Design review of the part built by this model. Coordinates are the model's own, in mm. Face numbers are marked on the shaded views. A direction names the side the tool comes from. Coordinates: 2 decimals unless noted, no trailing zeros. Loops run counter-clockwise (first coordinate to the right, second up) from the corner with the lowest first, then second, coordinate; pieces in that order, holes last. Notation, with made-up numbers: M 81.25,-26.5 L 128.25,-26.5 A30 cw 128.25,2.5 Z; hole C -39.5,48.5 d1. An arc over 180 degrees is marked long. One line per item, written item: value.
Autodesk Fusion 360 part; units mm, degrees
sketch "Sketch1" plane through (0, 0, 0) normal (0, 1, 0) x (1, 0, 0)
  line L0 (60, 15) -> (-60, 15)
  line L1 (-60, 15) -> (-60, -15)
  line L2 (-60, -15) -> (60, -15)
  line L3 (60, -15) -> (60, 15)
  line L4 (60, 15) -> (-60, -15) construction
  line L5 (-60, 15) -> (60, -15) construction
  line L6 (0, -15) -> (0, -60)
  line L7 (40, -15) -> (-40, -15)
  line L8 (-40, -15) -> (-40, -60)
  line L9 (-40, -60) -> (40, -60)
  line L10 (40, -60) -> (40, -15)
  line L11 (40, -15) -> (-40, -60) construction
  line L12 (-40, -15) -> (40, -60) construction
  line L13 (20, -40) -> (-20, -40)
  line L14 (-20, -40) -> (-20, -80)
  line L15 (-20, -80) -> (20, -80)
  line L16 (20, -80) -> (20, -40)
  line L17 (20, -40) -> (-20, -80) construction
  line L18 (-20, -40) -> (20, -80) construction
  point P0 (0, -37.5)
  point P1 (0, -60)
  dimension "d1" = 120
  dimension "d2" = 30
  dimension "d3" = 45
  dimension "d4" = 80
  dimension "d5" = 40
  dimension "d6" = 40
extrude "Extrude1" add sketch "Sketch1" along normal blind 80 contours L0 L1 L2 L3 L7 | L2 L6 L7 L9 L10 L13 L16 | L2 L6 L7 L8 L9 L13 L14
sketch "Sketch2" plane through (40, 0, 0) normal (1, 0, 0) x (0, 1, 0)
  line L0 (0, 60) -> (0, 15)
  line L1 (0, 15) -> (80, 15)
  line L2 (80, 15) -> (80, 60)
  line L3 (80, 60) -> (0, 60)
  circle A0 centre (40, 60) radius 15
  dimension "d9" = 30
extrude "Extrude2" cut sketch "Sketch2" against normal blind 100 contours L3 A0 | L3 A0
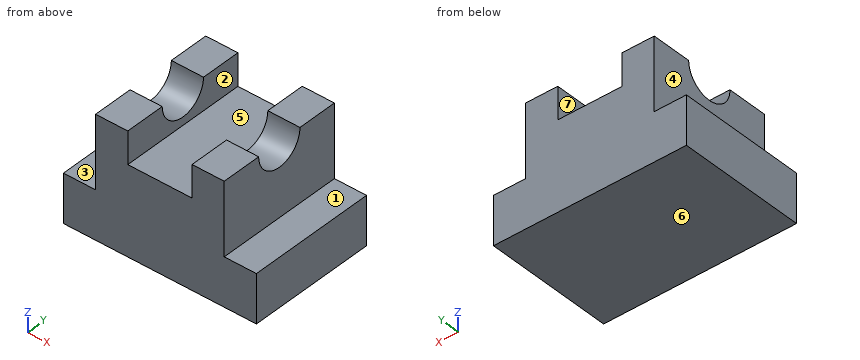
(1) We need section C-C on x = -6.5. State the section outline as (y, z) points.
Reply:
outline: M 0,-15 L 80,-15 L 80,40 L 0,40 Z
(2) Tool access review of the marked faces 1, 2 and 3: name each direction out of +Z, -Z, +X, -X, +Y, -Y from which nothing blocks a thin tool from reaching the whole face with its end or side.
Reply:
face 1: +Z, +X, +Y, -Y
face 2: +Z, +Y, -Y
face 3: +Z, -X, +Y, -Y
(3) Insertion check: pin 1 (10 mm diameter, centred on y = 51, z = 49, fed in from +X); pin 2 (22 mm diameter, centred on y = 31, z = 49, fed in from -X); pin 3 (3 mm diameter, centred on x = -9.5, y = 40, fed in from +Z). Each pin has a flat end and moves straight along its axis. Give the tip position at first contact, or say it passes through.
Reply:
pin 1: stops at x = 40
pin 2: stops at x = -40
pin 3: stops at z = 40
(4) Mouldability with a two-part tool opening along X and no side actions: class the marked faces 4, 5, 6 and 7 as released by +X, released by -X, zero draft, split by the parting line, or undercut.
Reply:
face 4: released by -X
face 5: undercut
face 6: zero draft
face 7: undercut
(5) We need section A-A on z = 50. State the section outline as (x, y) points.
Reply:
outline: M -40,0 L -20,0 L -20,28.82 L -40,28.82 Z; M -40,51.18 L -20,51.18 L -20,80 L -40,80 Z; M 20,0 L 40,0 L 40,28.82 L 20,28.82 Z; M 20,51.18 L 40,51.18 L 40,80 L 20,80 Z
(6) To check wall thickness, follow line 1 along X through (y, z) = (23, 50); line 2 along Z through (x, y) = (-44.5, 14); line 3 along X through (y, z) = (47, 30). State the ranges of each line that lie inside material, in increasing order. Write a range as [from, to].
Reply:
line 1: x = [-40, -20], [20, 40]
line 2: z = [-15, 15]
line 3: x = [-40, 40]
(7) We need section D-D on z = 23.5. State the section outline as (x, y) points, then the cut area to 3 significant figures.
Reply:
outline: M -40,0 L 40,0 L 40,80 L -40,80 Z
area: 6,400 mm2
(8) We need section B-B on y = 40. State the section outline as (x, z) points, then the cut area to 3 significant figures.
Reply:
outline: M -60,-15 L 60,-15 L 60,15 L 40,15 L 40,45 L 20,45 L 20,40 L -20,40 L -20,45 L -40,45 L -40,15 L -60,15 Z
area: 5,800 mm2
